The listing builds one solid part. Answer for the finished solid, in the listing's coordinates (mm). A direction names the side the tool comes from. Coordinates: 2 decimals unless noted, no trailing zeros. Order: outer loops, then holes, each group sorted by start corner. A loop starts at its lowest first (then second) coordinate and runs counter-clockwise, first axis right, second up. Notation, with made-up numbers: (64, 85.5) -> (90, 85.5) arc R23 ccw to (90, 99.5) -> close; hole circle Ø4 at (-16.5, -32). An arc over 180 degrees is marked (long way). Answer in a Markdown table with one row per item.
```python
from build123d import *

# Parameters (mm, degrees)
SKETCH_W        = 55
SKETCH_H        = 55
PAD_DEPTH       = 70
SKETCH001_W     = 46
SKETCH001_H     = 46
POCKET_DEPTH    = 70
POCKET001_DEPTH = 70
FILLET_R        = 4
FILLET001_R     = 7


with BuildPart() as part:
    # Sketch → Pad (new body)
    with BuildSketch(Plane.XY):
        Rectangle(SKETCH_W, SKETCH_H)
    extrude(amount=PAD_DEPTH)

    # Sketch001 → Pocket (cut)
    with BuildSketch(Plane.XY):
        Rectangle(SKETCH001_W, SKETCH001_H)
    extrude(amount=POCKET_DEPTH, mode=Mode.SUBTRACT)

    # Sketch002 (on Face5 of Pocket) → Pocket001 (cut)
    with BuildSketch(Plane.XY.offset(70)):
        Polygon((23, -23), (-17, -23), (-17, -27.5), (27.5, -27.5), (27.5, 17), (23, 17), align=None)
    extrude(amount=-POCKET001_DEPTH, mode=Mode.SUBTRACT)

    # Fillet
    fillet_edges = [part.edges().sort_by_distance(p)[0] for p in [
        (-23, -23, 35),
        (-23, 23, 35),
        (23, 23, 35),
    ]]
    fillet(fillet_edges, radius=FILLET_R)

    # Fillet001
    fillet001_edges = [part.edges().sort_by_distance(p)[0] for p in [
        (-27.5, -27.5, 35),
        (-27.5, 27.5, 35),
        (27.5, 27.5, 35),
    ]]
    fillet(fillet001_edges, radius=FILLET001_R)


solid = part.part
```
(1) For a pull along X with two mould halves and no side action, classify faces 6 (the flat face through (-27.5, 0, 35)), 7 (the flat face through (0, 23, 35)), 8 (the flat face through (-17, -25, 35)) as released by +X, released by -X, zero draft, split by the parting line, or undercut.
Check values:
| item | result |
|---|---|
| face 6 | released by -X |
| face 7 | undercut |
| face 8 | released by +X |
(2) Flat-ended cylindrical pins translate along their axes: pin 1 (3 mm diameter, centred on x = -15, z = 54.5, fed in from -Y); pin 2 (3.5 mm diameter, centred on y = -24.5, z = 51, fed in from +X); pin 3 (1 mm diameter, centred on x = 21.5, z = 29.5, fed in from +Y); pin 4 (12 mm diameter, centred on y = -21.5, z = 15, fed in from -X). Find the tip coordinate at first contact, or state that the pin passes through.
Check values:
| item | result |
|---|---|
| pin 1 | y = 23 |
| pin 2 | x = -17 |
| pin 3 | y = 27.48 |
| pin 4 | x = -27.5 |
(3) A cutting plane is placed at C-C, the plane y = -8.5. Determine the outline of the cut face in (x, z), then the cut area to 3 significant figures.
Check values:
| item | result |
|---|---|
| outline | (-27.5, 0) -> (-23, 0) -> (-23, 70) -> (-27.5, 70) -> close |
| area | 315 mm² |
(4) Which of the six approach directions +Z, -Z, +X, -X, +Y, -Y give full straight-line access (tool end or side, diameter ignored) to faces 1 (the flat face through (27.5, 19, 35)), 2 (the cylindrical face through (21.859, 21.797, 35.49)), 3 (the flat face through (-18, -23, 35)), 4 (the flat face through (25, 17, 35)), 5 (the cylindrical face through (-21.797, 21.859, 35.49))?
Check values:
| item | result |
|---|---|
| face 1 | +Z, -Z, +X, +Y, -Y |
| face 2 | +Z, -Z, -Y |
| face 3 | +Z, -Z, +X |
| face 4 | +Z, -Z, +X, -Y |
| face 5 | +Z, -Z |
(5) Find the intervals of material crossed by line 1 along X through (y, z) = (4.5, 47); line 2 along Y through (x, z) = (13.5, 66.5); line 3 along X through (y, z) = (20.5, 3), in increasing order. Write a range as from..to.
Check values:
| item | result |
|---|---|
| line 1 | -27.5..-23 |
| line 2 | 23..27.5 |
| line 3 | -27.5..-22.71, 22.71..27.5 |
(6) A cutting plane is placed at A-A, the plane z = 16. Determine the outline of the cut face in (x, y).
Check values:
| item | result |
|---|---|
| outline | (-27.5, -20.5) arc R7 ccw to (-20.5, -27.5) -> (-17, -27.5) -> (-17, -23) -> (-19, -23) arc R4 cw to (-23, -19) -> (-23, 19) arc R4 cw to (-19, 23) -> (19, 23) arc R4 cw to (23, 19) -> (23, 17) -> (27.5, 17) -> (27.5, 20.5) arc R7 ccw to (20.5, 27.5) -> (-20.5, 27.5) arc R7 ccw to (-27.5, 20.5) -> close |
(7) A cutting plane is placed at B-B, the plane x = 8.5. Determine the outline of the cut face in (y, z).
Check values:
| item | result |
|---|---|
| outline | (23, 0) -> (27.5, 0) -> (27.5, 70) -> (23, 70) -> close |
